Autodesk Inventor part; units mm, degrees
ref_plane "YZ Plane" through (0, 0, 0) normal (1, 0, 0) x (0, 1, 0)
ref_plane "XZ Plane" through (0, 0, 0) normal (0, 1, 0) x (-1, 0, 0)
ref_plane "XY Plane" through (0, 0, 0) normal (0, 0, 1) x (1, 0, 0)
sketch "Skizze1" plane through (0, 0, 0) normal (0, 0, 1) x (1, 0, 0)
  circle A0 centre (-57.772, 35) radius 20 construction
  circle A1 centre (57.772, 35) radius 20 construction
  circle A2 centre (35, -57.772) radius 20 construction
  circle A3 centre (-35, -57.772) radius 20 construction
  line L0 (0, 81.5544) -> (0, -104.3264) construction
  line L1 (-108.8808, 0) -> (108.8808, 0) construction
  circle A4 centre (0, 0) radius 25 construction
  line L2 (10, 25) -> (10, -23.5147)
  circle A5 centre (-6, -2.5) radius 6 construction
  line L3 (0, 3.5) -> (-21.5, 25)
  line L4 (0, -6.5) -> (-10, -16.5)
  line L5 (-10, -16.5) -> (-10, -23.5147)
  line L6 (-10, -23.5147) -> (-31.444, -44.9587)
  line L7 (-31.444, -44.9587) -> (-27.2013, -49.2013)
  line L8 (-27.2013, -49.2013) -> (0, -22)
  line L9 (0, -22) -> (27.2013, -49.2013)
  line L10 (27.2013, -49.2013) -> (31.444, -44.9587)
  line L11 (31.444, -44.9587) -> (10, -23.5147)
  line L12 (0, -6.5) -> (0, 3.5)
  line L13 (10, 25) -> (47.5055, 25)
  line L14 (47.5055, 25) -> (47.5055, 31)
  line L15 (-10, 31) -> (-47.5055, 31)
  line L16 (-47.5055, 31) -> (-47.5055, 25)
  line L17 (-47.5055, 25) -> (-21.5, 25)
  line L18 (-10, 31) -> (-10, 45)
  line L19 (-10, 45) -> (6, 45)
  line L20 (6, 45) -> (6, 31)
  line L21 (6, 31) -> (47.5055, 31)
  line L22 (-61.4468, -24.6516) -> (-51.4468, -24.6516) construction
  line L23 (-51.4468, -24.6516) -> (-56.4468, -27.5384) construction
  line L24 (-56.4468, -27.5384) -> (-61.4468, -24.6516) construction
  line L25 (-56.4468, -27.5384) -> (-56.4468, -24.6516) construction
  circle A6 centre (-27.2013, -44.9587) radius 3 construction
  circle A7 centre (-27.2013, -44.9587) radius 5 construction
  circle A8 centre (-44.5055, 28) radius 3 construction
  circle A9 centre (-44.5055, 28) radius 5 construction
  circle A10 centre (-5, -17) radius 1.05
  circle A11 centre (-5, 42) radius 1.05
  dimension "d0" = 35
  dimension "d1" = 57.772
  dimension "d2" = 40
  dimension "d3" = 57.772
  dimension "d4" = 35
  dimension "d5" = 40
  dimension "d6" = 50
  dimension "d7" = 10
  dimension "d9" = 6
  dimension "d10" = 2.5
  dimension "d11" = 12
  dimension "d12" = 6
  dimension "d13" = 6
  dimension "d14" = 4
  dimension "d15" = 10
  dimension "d16" = 6
  dimension "d20" = 31
  dimension "d21" = 10
  dimension "d22" = 120
  dimension "d23" = 2.8868
  dimension "d24" = 10
  dimension "d25" = 10
  dimension "d26" = 22
  dimension "d27" = 2.1
  dimension "d28" = 5
  dimension "d29" = 17
  dimension "d30" = 5
  dimension "d31" = 42
  dimension "d32" = 45
  dimension "d33" = 6
extrude "Extrusion1" add sketch "Skizze1" along normal blind 1.6
equation "\"d3\" = d1"
equation "\"d4\" = d0"
equation "\"d5\" = d2"
equation "\"d25\" = d24"
properties part number "Color Detect PCB" material "Phenolharz"
Work out the finished part from the listing and answer in its coordinate system (mm). A direction names the side the tool comes from. Coordinates: 2 decimals unless noted, no trailing zeros. Write each loop counter-clockwise with the first axis right and the second up, starting at its lowest first coordinate (ties: lowest second). Pieces come first, ordered by that corner, then holes. Notation, with made-up numbers: M 61.5,37 L 116.5,37 A26 ccw 116.5,76 Z; hole C 82,78.5 d3. An arc over 180 degrees is marked long. Use one line per item in the form item = value. Start each with the question number.
1. The part is cut by section B-B (x = 15.5). Give the vertices of the cut face in (y, z).
2. The part is cut by section A-A (z = 1.2). Give the vertices of the cut face in (x, y).
3. The part is cut by section C-C (x = -41). Give the vertices of the cut face in (y, z).
4. The mould has two halves that part along Y. Classify faces 6 (the face through (-10.6, 14.1, 0.8)), 7 (the face through (0, 9, 0)), 8 (the face through (13, -35, 1)): released by +Y, released by -Y, zero draft, split by the parting line, or undercut.
5. A tool of negligible diameter and unlimited length cuts with its end or side. For faces 1 (the face through (20.872, -34.387, 0.789)), 2 (the face through (-20.572, -34.087, 0.789)), 3 (the face through (-5.228, -15.975, 0.789)), 4 (the face through (-14, -36, 1)), 5 (the face through (0, 9, 1.6)), from which of +Z, -Z, +X, -X, +Y, -Y can it reach the whole face along a straight path? Write none if from no direction.
6. Each of these flat-tipped pins is pushed along its axis until it touches: P1, Ø1.7, axis at x = -5, y = 42, coming from the -Z side; P2, Ø0.5, axis at x = 30.5, z = 1, coming from the -Y side; P3, Ø0.8, axis at x = -33, z = 0.5, coming from the +Y side; P4, Ø0.5, axis at y = -7, z = 0.5, coming from the +X side. Where does it stop, or does it pass through?
7. Straight lines are drawn through the part: probe 1 along Y at (x, z) = (-5, 1.2); probe 2 along Y at (x, z) = (20, 0.65); probe 3 along Y at (x, z) = (-18, 0.15). For each, find the intervals that lie inside material, in ascending order. Write a range as from..to.
8. The part is cut by section D-D (y = -2.5). Give the vertices of the cut face in (x, z), plus the area to 3 significant figures.
Evaluation:
q1.outline = M -37.5,0 L -29.01,0 L -29.01,1.6 L -37.5,1.6 Z; M 25,0 L 31,0 L 31,1.6 L 25,1.6 Z
q2.outline = M -47.51,25 L -21.5,25 L 0,3.5 L 0,-6.5 L -10,-16.5 L -10,-23.51 L -31.44,-44.96 L -27.2,-49.2 L 0,-22 L 27.2,-49.2 L 31.44,-44.96 L 10,-23.51 L 10,25 L 47.51,25 L 47.51,31 L 6,31 L 6,45 L -10,45 L -10,31 L -47.51,31 Z; hole C -5,-17 d2.1; hole C -5,42 d2.1
q3.outline = M 25,0 L 31,0 L 31,1.6 L 25,1.6 Z
q4.face_6 = undercut
q4.face_7 = zero draft
q4.face_8 = released by -Y
q5.face_1 = +Z, -Z, +X
q5.face_2 = +Z, -Z, -X
q5.face_3 = +Z, -Z
q5.face_4 = +Z, -Z, -Y
q5.face_5 = +Z, +X, -X, +Y, -Y
q6.P1 = through
q6.P2 = -46.15
q6.P3 = 31
q6.P4 = 10
q7.probe_1 = -27..-18.05, -15.95..-11.5, 8.5..40.95, 43.05..45
q7.probe_2 = -42..-33.51, 25..31
q7.probe_3 = -40..-31.51, 21.5..31
q8.outline = M 0,0 L 10,0 L 10,1.6 L 0,1.6 Z
q8.area = 16.0 mm^2
